Check sheet for the modelled part. Datum: model origin and axes. Units: mm. A direction names the side the tool comes from. Round coordinates to 2 decimals unless told otherwise and drop trailing zeros. Write each loop counter-clockwise with the first axis right and the second up, starting at its lowest first coordinate (ties: lowest second). Pieces come first, ordered by that corner, then holes.
Item 1: Cross-section at B-B on x = 0. Enter the section's corners in (y, z), plus the area to 3 significant figures.
Item 2: Cross-section at A-A on y = 0. Count the separate pieces of the cut face and the enclosed holes in it, plus the area to 3 significant figures.
Item 3: Cross-section at D-D on z = -44. Enter the section's corners in (x, y).
Item 4: Material ranges on line 1 (Z direction, x = 119, y = -97); line 2 (Z direction, x = 42.5, y = -151.5); line 3 (X direction, y = 78.5, z = 58), recorded low to high.
Item 5: Tool access check on faces 4 (the cylindrical face through (128.615, 100.088, -6.409)), 5 (the flat face through (126.697, 77.325, -6.409)), 6 (the cylindrical face through (141.426, -156.025, 52.297)), 7 (the cylindrical face through (133, 145, -52)), 8 (the cylindrical face through (141.426, -156.025, -52.297)). Record the directions out of +Z, -Z, +X, -X, +Y, -Y that give a thin tool (end or side, any length) a straight path to the whole face; none if there is none.
Item 6: Cross-section at C-C on z = 19. Enter the section's corners in (x, y) (3 decimals).
Item 7: Go/stop test with flat-tipped pins: pin 1 Ø6 at (y, z) = (114, -15.5) entering from +X; pin 2 Ø5 at (x, z) = (88.5, 18) entering from -Y; pin 3 Ø4 at (y, z) = (98, 44) entering from +X. Record where each tip stops, or that it passes through.
Item 8: Release check for a two-part mould opening along X. For faces 1 (the cylindrical face through (142.926, 6.218, -6.409)), 2 (the cylindrical face through (-1.302, -183.282, 4.93)), 3 (the cylindrical face through (122.945, 188.71, -25.325)) record: +X half, -X half, draft (parallel to the pull), parting line (faces both ways), or undercut.
from build123d import *

# Parameters (mm, degrees)
SKETCH2_R                = 210
SKETCH2_R_2              = 135
BOSS_EXTRUDE1_DEPTH      = 10
SKETCH3_R                = 10
CUT_EXTRUDE1_DEPTH       = 10
CUT_EXTRUDE1_DEPTH_BACK  = 10
BOSS_EXTRUDE2_DEPTH      = 25
BOSS_EXTRUDE3_DEPTH      = 25
BOSS_EXTRUDE4_DEPTH      = 67
BOSS_EXTRUDE4_DEPTH_BACK = 67


with BuildPart() as part:
    # Sketch2 → Boss-Extrude1 (new body)
    with BuildSketch(Plane.XY):
        Circle(SKETCH2_R)
        Circle(SKETCH2_R_2, mode=Mode.SUBTRACT)
    extrude(amount=BOSS_EXTRUDE1_DEPTH)

    # Sketch3 → Cut-Extrude1 (cut, two sides)
    with BuildSketch(Plane.XY) as cut_extrude1_sk:
        with Locations((0, 193.197162002)):
            Circle(SKETCH3_R)
        with Locations((37.071880295, 173.226532384)):
            Circle(SKETCH3_R)
        with Locations((100.540875426, 145.853653362)):
            Circle(SKETCH3_R)
        with Locations((148.703433678, 96.275877783)):
            Circle(SKETCH3_R)
        with Locations((174.227242153, 32.040972553)):
            Circle(SKETCH3_R)
        with Locations((173.226532384, -37.071880295)):
            Circle(SKETCH3_R)
        with Locations((145.853653362, -100.540875426)):
            Circle(SKETCH3_R)
        with Locations((96.275877783, -148.703433678)):
            Circle(SKETCH3_R)
        with Locations((32.040972554, -174.227242153)):
            Circle(SKETCH3_R)
        with Locations((-37.071880295, -173.226532384)):
            Circle(SKETCH3_R)
        with Locations((-100.540875426, -145.853653362)):
            Circle(SKETCH3_R)
        with Locations((-148.703433678, -96.275877783)):
            Circle(SKETCH3_R)
        with Locations((-174.227242153, -32.040972553)):
            Circle(SKETCH3_R)
        with Locations((-173.226532384, 37.071880295)):
            Circle(SKETCH3_R)
        with Locations((-145.853653362, 100.540875426)):
            Circle(SKETCH3_R)
        with Locations((-96.275877783, 148.703433678)):
            Circle(SKETCH3_R)
        with Locations((-32.040972553, 174.227242153)):
            Circle(SKETCH3_R)
        with Locations((73.933353078, 178.490903713)):
            Circle(SKETCH3_R)
        with Locations((136.611023358, 136.611023358)):
            Circle(SKETCH3_R)
        with Locations((178.490903713, 73.933353078)):
            Circle(SKETCH3_R)
        with Locations((193.197162002, 0)):
            Circle(SKETCH3_R)
        with Locations((178.490903713, -73.933353078)):
            Circle(SKETCH3_R)
        with Locations((136.611023358, -136.611023358)):
            Circle(SKETCH3_R)
        with Locations((73.933353078, -178.490903713)):
            Circle(SKETCH3_R)
        with Locations((0, -193.197162002)):
            Circle(SKETCH3_R)
        with Locations((-73.933353078, -178.490903713)):
            Circle(SKETCH3_R)
        with Locations((-136.611023358, -136.611023358)):
            Circle(SKETCH3_R)
        with Locations((-178.490903713, -73.933353078)):
            Circle(SKETCH3_R)
        with Locations((-193.197162002, 0)):
            Circle(SKETCH3_R)
        with Locations((-178.490903713, 73.933353078)):
            Circle(SKETCH3_R)
        with Locations((-136.611023358, 136.611023358)):
            Circle(SKETCH3_R)
        with Locations((-73.933353078, 178.490903713)):
            Circle(SKETCH3_R)
        with Locations((0, 156.410432221)):
            Circle(SKETCH3_R)
        with Locations((63.617854144, 142.888039883)):
            Circle(SKETCH3_R)
        with Locations((116.235603356, 104.659007353)):
            Circle(SKETCH3_R)
        with Locations((148.75516078, 48.333481654)):
            Circle(SKETCH3_R)
        with Locations((155.553599508, -16.349342119)):
            Circle(SKETCH3_R)
        with Locations((135.45540772, -78.20521611)):
            Circle(SKETCH3_R)
        with Locations((91.935745364, -126.538697764)):
            Circle(SKETCH3_R)
        with Locations((32.519557425, -152.992489006)):
            Circle(SKETCH3_R)
        with Locations((-32.519557425, -152.992489006)):
            Circle(SKETCH3_R)
        with Locations((-91.935745364, -126.538697764)):
            Circle(SKETCH3_R)
        with Locations((-135.45540772, -78.20521611)):
            Circle(SKETCH3_R)
        with Locations((-155.553599508, -16.349342119)):
            Circle(SKETCH3_R)
        with Locations((-148.75516078, 48.333481654)):
            Circle(SKETCH3_R)
        with Locations((-116.235603356, 104.659007353)):
            Circle(SKETCH3_R)
        with Locations((-63.617854143, 142.888039883)):
            Circle(SKETCH3_R)
    extrude(amount=CUT_EXTRUDE1_DEPTH, mode=Mode.SUBTRACT)
    extrude(cut_extrude1_sk.sketch, amount=-CUT_EXTRUDE1_DEPTH_BACK, mode=Mode.SUBTRACT)



with BuildPart() as body_2:
    # Sketch4 → Boss-Extrude2 (new body)
    with BuildSketch(Plane.XY.offset(13)):
        with BuildLine():
            Line((89.699423037, 192.385548243), (89.699423037, 99.043714713))
            ThreePointArc((89.699423037, 99.043714713), (90.387508707, 95.592326562), (92.346551963, 92.668683018))
            ThreePointArc((92.346551963, 92.668683018), (130.825725573, 0), (92.346551963, -92.668683018))
            ThreePointArc((92.346551963, -92.668683018), (90.387508707, -95.592326562), (89.699423037, -99.043714713))
            Line((89.699423037, -99.043714713), (89.699423037, -192.385548243))
            ThreePointArc((89.699423037, -192.385548243), (94.00759833, -200.065833454), (102.807596575, -200.393226445))
            ThreePointArc((102.807596575, -200.393226445), (122.675577525, -188.885017398), (141.268660314, -175.413832783))
            ThreePointArc((141.268660314, -175.413832783), (149.513380795, -156.502698139), (168.781213285, -149.129974051))
            ThreePointArc((168.781213285, -149.129974051), (181.513487561, -133.340545041), (192.773608207, -116.469665997))
            ThreePointArc((192.773608207, -116.469665997), (195.045606898, -92.634226865), (212.083561399, -75.811675242))
            ThreePointArc((212.083561399, -75.811675242), (225.226213214, 0), (212.083561399, 75.811675242))
            ThreePointArc((212.083561399, 75.811675242), (195.045606898, 92.634226865), (192.773608207, 116.469665997))
            ThreePointArc((192.773608207, 116.469665997), (181.513487561, 133.340545041), (168.781213285, 149.129974051))
            ThreePointArc((168.781213285, 149.129974051), (149.513380795, 156.502698139), (141.268660314, 175.413832783))
            ThreePointArc((141.268660314, 175.413832783), (122.675577525, 188.885017398), (102.807596575, 200.393226445))
            ThreePointArc((102.807596575, 200.393226445), (94.00759833, 200.065833454), (89.699423037, 192.385548243))
        make_face()
    extrude(amount=BOSS_EXTRUDE2_DEPTH)


with BuildPart() as body_3:
    # Sketch6 → Boss-Extrude3 (new body)
    with BuildSketch(Plane(origin=(0, 0, -13), x_dir=(-1, 0, 0), z_dir=(0, 0, -1))):
        with BuildLine():
            Line((-89.699423037, -99.043714713), (-89.699423037, -192.385548243))
            ThreePointArc((-89.699423037, -192.385548243), (-94.00759833, -200.065833454), (-102.807596575, -200.393226445))
            ThreePointArc((-102.807596575, -200.393226445), (-122.675577525, -188.885017398), (-141.268660314, -175.413832783))
            ThreePointArc((-141.268660314, -175.413832783), (-149.513380795, -156.502698139), (-168.781213285, -149.129974051))
            ThreePointArc((-168.781213285, -149.129974051), (-181.513487561, -133.340545041), (-192.773608207, -116.469665997))
            ThreePointArc((-192.773608207, -116.469665997), (-195.045606898, -92.634226865), (-212.083561399, -75.811675242))
            ThreePointArc((-212.083561399, -75.811675242), (-225.226213214, 0), (-212.083561399, 75.811675242))
            ThreePointArc((-212.083561399, 75.811675242), (-195.045606898, 92.634226865), (-192.773608207, 116.469665997))
            ThreePointArc((-192.773608207, 116.469665997), (-181.513487561, 133.340545041), (-168.781213285, 149.129974051))
            ThreePointArc((-168.781213285, 149.129974051), (-149.513380795, 156.502698139), (-141.268660314, 175.413832783))
            ThreePointArc((-141.268660314, 175.413832783), (-122.675577525, 188.885017398), (-102.807596575, 200.393226445))
            ThreePointArc((-102.807596575, 200.393226445), (-94.00759833, 200.065833454), (-89.699423037, 192.385548243))
            Line((-89.699423037, 192.385548243), (-89.699423037, 99.043714713))
            ThreePointArc((-89.699423037, 99.043714713), (-90.387508707, 95.592326562), (-92.346551963, 92.668683018))
            ThreePointArc((-92.346551963, 92.668683018), (-130.825725573, 0), (-92.346551963, -92.668683018))
            ThreePointArc((-92.346551963, -92.668683018), (-90.387508707, -95.592326562), (-89.699423037, -99.043714713))
        make_face()
    extrude(amount=BOSS_EXTRUDE3_DEPTH)


with BuildPart() as part_1:
    add(part.part)

    add(body_2.part)  # Boss-Extrude4 merges body 2

    add(body_3.part)  # Boss-Extrude4 merges body 3
    # Sketch7 → Boss-Extrude4 (add, two sides)
    with BuildSketch(Plane.XY) as boss_extrude4_sk:
        with BuildLine():
            Line((124.797572435, 128.173439312), (125.442001569, 110.919091112))
            ThreePointArc((125.442001569, 110.919091112), (128.621769694, 99.926736137), (126.270819, 88.727815472))
            Line((126.270819, 88.727815472), (127.134644848, 65.599202612))
            ThreePointArc((127.134644848, 65.599202612), (142.961406409, 5.33943643), (131.673727115, -55.933021476))
            Line((131.673727115, -55.933021476), (132.528568771, -78.821085957))
            ThreePointArc((132.528568771, -78.821085957), (140.793126639, -98.20534295), (133.997533992, -118.152078436))
            Line((133.997533992, -118.152078436), (134.440437213, -130.010645939))
            ThreePointArc((134.440437213, -130.010645939), (138.90259856, -139.536805522), (135.321811068, -149.428042109))
            ThreePointArc((135.321811068, -149.428042109), (141.553905611, -156.063570567), (150.388109377, -153.866735539))
            ThreePointArc((150.388109377, -153.866735539), (215.00481878, 8.030171155), (138.491666876, 164.656047424))
            ThreePointArc((138.491666876, 164.656047424), (131.044013158, 166.615042764), (124.807721177, 162.096871567))
            ThreePointArc((124.807721177, 162.096871567), (132.998470182, 145.132703527), (124.797572435, 128.173439312))
        make_face()
    extrude(amount=BOSS_EXTRUDE4_DEPTH)
    extrude(boss_extrude4_sk.sketch, amount=-BOSS_EXTRUDE4_DEPTH_BACK)


solid = part_1.part
Response values:
1. outline: (-210, 0) - (-203.2, 0) - (-203.2, 10) - (-210, 10) - close; (-183.2, 0) - (-135, 0) - (-135, 10) - (-183.2, 10) - close; (135, 0) - (146.41, 0) - (146.41, 10) - (135, 10) - close; (166.41, 0) - (183.2, 0) - (183.2, 10) - (166.41, 10) - close; (203.2, 0) - (210, 0) - (210, 10) - (203.2, 10) - close
1. area: 900 mm2
2. separate pieces: 3
2. enclosed holes: 0
2. area: 11,400 mm2
3. outline: (124.8, 128.17) - (125.44, 110.92) arc R23.66 cw to (126.27, 88.73) - (127.13, 65.6) arc R143.06 cw to (131.67, -55.93) - (132.53, -78.82) arc R29.46 cw to (134, -118.15) - (134.44, -130.01) arc R13.74 cw to (135.32, -149.43) arc R9 ccw to (150.39, -153.87) arc R215.15 ccw to (138.49, 164.66) arc R9 ccw to (124.81, 162.1) arc R21.65 cw to start
4. line 1: z = -38 to -13, 0 to 10, 13 to 38
4. line 2: z = 0 to 10
4. line 3: x = 126.65 to 200.32
5. face 4: -X
5. face 5: -X, -Y
5. face 6: +Z, -Y
5. face 7: -Z, -X
5. face 8: -Z, -Y
6. outline: (89.699, -192.386) arc R9 ccw to (102.808, -200.393) arc R225.226 ccw to (141.269, -175.414) arc R26.671 cw to (168.781, -149.13) arc R225.226 ccw to (192.774, -116.47) arc R35.071 cw to (212.084, -75.812) arc R225.226 ccw to (212.084, 75.812) arc R35.071 cw to (192.774, 116.47) arc R225.226 ccw to (168.781, 149.13) arc R26.671 cw to (141.269, 175.414) arc R225.226 ccw to (102.808, 200.393) arc R9 ccw to (89.699, 192.386) - (89.699, 99.044) arc R9 ccw to (92.347, 92.669) arc R130.826 cw to (92.347, -92.669) arc R9 ccw to (89.699, -99.044) - close
7. pin 1: stops at x = 192.77
7. pin 2: stops at y = -197.05
7. pin 3: stops at x = 192.55
8. face 1: -X half
8. face 2: undercut
8. face 3: +X half
